```python
from build123d import *

# Parameters (mm, degrees)
SKETCH5_W           = 127
SKETCH5_H           = 127
SKETCH5_W_2         = 20.32
SKETCH5_H_2         = 20.32
BOSS_EXTRUDE1_DEPTH = 304.8
SKETCH6_R           = 44.45
CUT_EXTRUDE1_DEPTH  = 203.2
SKETCH5_3_W         = 20.32
SKETCH5_3_H         = 20.32
CUT_EXTRUDE2_DEPTH  = 25.4
CUT_EXTRUDE3_START  = -76.2
CUT_EXTRUDE3_DEPTH  = 76.2
SKETCH9_R           = 7.62
CUT_EXTRUDE4_DEPTH  = 56.642


with BuildPart() as part:
    # Sketch5 → Boss-Extrude1 (new body)
    # profile 1 of 5: a face of its own
    with BuildSketch(Plane(origin=(0, 0, 0), x_dir=(1, 0, 0), z_dir=(0, 1, 0))):
        with Locations((63.5, 63.5)):
            Rectangle(SKETCH5_W, SKETCH5_H)
        with Locations((16.51, 15.457317153)):
            Rectangle(SKETCH5_W_2, SKETCH5_H_2, mode=Mode.SUBTRACT)
        with Locations((110.49, 15.457317153)):
            Rectangle(SKETCH5_W_2, SKETCH5_H_2, mode=Mode.SUBTRACT)
        with Locations((110.49, 110.49)):
            Rectangle(SKETCH5_W_2, SKETCH5_H_2, mode=Mode.SUBTRACT)
        with Locations((16.51, 110.49)):
            Rectangle(SKETCH5_W_2, SKETCH5_H_2, mode=Mode.SUBTRACT)
    # profile 2 of 5: a face of its own
    with BuildSketch(Plane(origin=(0, 0, 0), x_dir=(1, 0, 0), z_dir=(0, 1, 0))):
        with Locations((110.49, 15.457317153)):
            Rectangle(SKETCH5_W_2, SKETCH5_H_2)
    # profile 3 of 5: a face of its own
    with BuildSketch(Plane(origin=(0, 0, 0), x_dir=(1, 0, 0), z_dir=(0, 1, 0))):
        with Locations((110.49, 110.49)):
            Rectangle(SKETCH5_W_2, SKETCH5_H_2)
    # profile 4 of 5: a face of its own
    with BuildSketch(Plane(origin=(0, 0, 0), x_dir=(1, 0, 0), z_dir=(0, 1, 0))):
        with Locations((16.51, 15.457317153)):
            Rectangle(SKETCH5_W_2, SKETCH5_H_2)
    # profile 5 of 5: a face of its own
    with BuildSketch(Plane(origin=(0, 0, 0), x_dir=(1, 0, 0), z_dir=(0, 1, 0))):
        with Locations((16.51, 110.49)):
            Rectangle(SKETCH5_W_2, SKETCH5_H_2)
    extrude(amount=BOSS_EXTRUDE1_DEPTH)

    # Sketch6 → Cut-Extrude1 (cut)
    with BuildSketch(Plane(origin=(0, 0, 0), x_dir=(1, 0, 0), z_dir=(0, 1, 0))):
        with Locations(Location((63.5, 63.5, 0), (0, 0, 270))):
            Circle(SKETCH6_R)
    extrude(amount=CUT_EXTRUDE1_DEPTH, mode=Mode.SUBTRACT)

    # Sketch5_3 → Cut-Extrude2 (cut)
    with BuildSketch(Plane(origin=(0, 0, 0), x_dir=(1, 0, 0), z_dir=(0, 1, 0))):
        with Locations((16.51, 15.457317153)):
            Rectangle(SKETCH5_3_W, SKETCH5_3_H)
        with Locations((110.49, 15.457317153)):
            Rectangle(SKETCH5_3_W, SKETCH5_3_H)
        with Locations((110.49, 110.49)):
            Rectangle(SKETCH5_3_W, SKETCH5_3_H)
        with Locations((16.51, 110.49)):
            Rectangle(SKETCH5_3_W, SKETCH5_3_H)
    extrude(amount=CUT_EXTRUDE2_DEPTH, mode=Mode.SUBTRACT)

    # Sketch7 → Cut-Extrude3 (cut)
    with BuildSketch(Plane(origin=(0, 297.18, 0), x_dir=(1, 0, 0), z_dir=(0, 1, 0)).offset(CUT_EXTRUDE3_START)):
        with BuildLine():
            Line((107.95, 63.5), (107.95, -124.596764807))
            Line((107.95, -124.596764807), (19.05, -124.596764807))
            Line((19.05, -124.596764807), (19.05, 63.5))
            ThreePointArc((19.05, 63.5), (63.5, 107.95), (107.95, 63.5))
        make_face()
    extrude(amount=CUT_EXTRUDE3_DEPTH, mode=Mode.SUBTRACT)

    # Sketch9 → Cut-Extrude4 (cut)
    with BuildSketch(Plane.XY):
        with Locations((63.5, 190.5)):
            Circle(SKETCH9_R)
        with Locations((63.5, 165.1)):
            Circle(SKETCH9_R)
    extrude(amount=-CUT_EXTRUDE4_DEPTH, mode=Mode.SUBTRACT)


solid = part.part
```
Build history of the part. All positions in model axes, mm. A direction names the side the tool comes from. Round coordinates to 2 decimals unless told otherwise and drop trailing zeros. Loops run counter-clockwise (first coordinate to the right, second up) from the corner with the lowest first, then second, coordinate; pieces in that order, holes last. Notation, with made-up numbers: M 59.25,-26.5 L 65.25,-26.5 A22 ccw 65.25,6.5 Z; hole C -5.5,5 d11. An arc over 180 degrees is marked long. Answer as CSV lines item,"result".
1. Cut at C-C on y = 250.5. Write the cut outline in (x, z), then the cut area to 3 significant figures.
Resolved:
outline,"M 0,-127 L 127,-127 L 127,0 L 107.95,0 L 107.95,-63.5 A44.45 cw 19.05,-63.5 L 19.05,0 L 0,0 Z"
area,"7,380 mm²"
2. 3-axis set-ups, long thin cutter, end or side, ignore diameter. For faces 4 (the flat face through (16, 13, -100.33)), 5 (the flat face through (127, 150, -63)), 6 (the flat face through (19.05, 259, -31)): which of +Z, -Z, +X, -X, +Y, -Y reach the whole face in a straight line?
Resolved:
face 4,"-Y"
face 5,"+Z, -Z, +X, +Y, -Y"
face 6,"+Z"
3. Two-plate mould, pull along Y, no slides. Class faces 1 (the flat face through (63, 150, -127)), 2 (the flat face through (48, 0, -107)), 3 (the cylindrical face through (62.508, 198.055, -9.716)): released by +Y, released by -Y, zero draft, split by the parting line, or undercut.
Resolved:
face 1,"zero draft"
face 2,"released by -Y"
face 3,"undercut"
4. Cut at D-D on x = 38. Write the cut outline in (y, z), then the cut area to 3 significant figures.
Resolved:
outline,"M 0,-127 L 304.8,-127 L 304.8,0 L 297.18,0 L 297.18,-99.91 L 220.98,-99.91 L 220.98,0 L 0,0 L 0,-27.09 L 203.2,-27.09 L 203.2,-99.91 L 0,-99.91 Z"
area,"16,300 mm²"
5. Cut at B-B on z = -94. Write the cut outline in (x, y) (3 decimals), then the cut area to 3 significant figures.
Resolved:
outline,"M 0,0 L 31.165,0 L 31.165,203.2 L 95.835,203.2 L 95.835,0 L 127,0 L 127,304.8 L 0,304.8 Z; hole M 31.165,220.98 L 95.835,220.98 L 95.835,297.18 L 31.165,297.18 Z"
area,"20,600 mm²"
6. Flat gauge pins, fed straight in: P1, Ø8, axis at x = 65.5, z = -97.5, coming from the -Y side; P2, Ø9, axis at x = 63.5, y = 165.1, coming from the +Z side; P3, Ø10, axis at x = 15, z = -111.5, coming from the -Y side. Where does each tip first touch, or does it go through?
Resolved:
P1,"stops at y = 203.2"
P2,"stops at z = -107.72"
P3,"stops at y = 25.4"
7. Wall check: probe 1 along Y at (x, z) = (63.5, -5.25); probe 2 along Y at (x, z) = (25, -17); probe 3 along Y at (x, z) = (58, -27.5). Give the ranges that are in metal, low to high. Write a range as [from, to].
Resolved:
probe 1,"y = [0, 157.48], [172.72, 182.88], [198.12, 220.98], [297.18, 304.8]"
probe 2,"y = [25.4, 220.98], [297.18, 304.8]"
probe 3,"y = [203.2, 220.98], [297.18, 304.8]"
8. Cut at A-A on y = 71. Write the cut outline in (x, z), then the cut area to 3 significant figures.
Resolved:
outline,"M 0,-127 L 127,-127 L 127,0 L 0,0 Z; hole C 63.5,-63.5 d88.9"
area,"9,920 mm²"
